```python
from build123d import *

# Parameters (mm, degrees)
SKETCH_1_R          = 15.75
SKETCH_1_R_2        = 1.6
EXTRUDE_1_DEPTH     = 3
EXTRUDE_2_DEPTH     = 3
SKETCH_3_W          = 20
SKETCH_3_H          = 31.5
EXTRUDE_3_DEPTH     = 5
SKETCH_4_R          = 1.25
CUT_EXTRUDE_1_DEPTH = 10


with BuildPart() as part:
    # 草图1 → 凸台-拉伸1 (new body)
    with BuildSketch(Plane(origin=(0, 0, 0), x_dir=(1, 0, 0), z_dir=(0, 1, 0))):
        Circle(SKETCH_1_R)
        with Locations((0, 8)):
            Circle(SKETCH_1_R_2, mode=Mode.SUBTRACT)
        with Locations((8, 0)):
            Circle(SKETCH_1_R_2, mode=Mode.SUBTRACT)
        with Locations((0, -8)):
            Circle(SKETCH_1_R_2, mode=Mode.SUBTRACT)
        with Locations((-8, 0)):
            Circle(SKETCH_1_R_2, mode=Mode.SUBTRACT)
    extrude(amount=EXTRUDE_1_DEPTH)

    # 草图2 → 凸台-拉伸2 (add)
    with BuildSketch(Plane.XZ):
        with BuildLine():
            Line((0, 15.75), (55, 15.75))
            Line((55, 15.75), (55, -15.75))
            Line((55, -15.75), (0, -15.75))
            ThreePointArc((0, -15.75), (15.75, 0), (0, 15.75))
        make_face()
    extrude(amount=-EXTRUDE_2_DEPTH)

    # 草图3 → 凸台-拉伸3 (add)
    with BuildSketch(Plane.XZ):
        with Locations((45, 0)):
            Rectangle(SKETCH_3_W, SKETCH_3_H)
    extrude(amount=-EXTRUDE_3_DEPTH)

    # 草图4 → 切除-拉伸1 (cut)
    with BuildSketch(Plane(origin=(0, 5, 0), x_dir=(1, 0, 0), z_dir=(0, 1, 0))):
        with Locations((45, 4.5)):
            Circle(SKETCH_4_R)
        with Locations((45, -4.5)):
            Circle(SKETCH_4_R)
    extrude(amount=-CUT_EXTRUDE_1_DEPTH, mode=Mode.SUBTRACT)


solid = part.part
```
Input: part model. Units: mm. Frame: model coordinates. A direction names the side the tool comes from. Coordinates: 2 decimals unless noted, no trailing zeros. Write each loop counter-clockwise with the first axis right and the second up, starting at its lowest first coordinate (ties: lowest second). Pieces come first, ordered by that corner, then holes.
1) Section D-D on z = 4.5. Output: boundary loops of the cut face in (x, y), and give its area (3 significant figures).
2) Set-up query: faces 5 (the flat face through (10, 3, 0)), 6 (the flat face through (33, 2, 15.75)). Return all of +Z, -Z, +X, -X, +Y, -Y with unobstructed straight access to the full face (end or side cutting, diameter ignored); none if empty.
3) Section B-B on y = 1.45. Output: boundary loops of the cut face in (x, z), and give its area (3 significant figures).
4) Section C-C on x = 8. Output: boundary loops of the cut face in (y, z), and give its area (3 significant figures).
5) Pin query (flat end, axial travel): pin 1 Ø3 at (x, z) = (45, -4.5) entering from +Y; pin 2 Ø4 at (x, z) = (0, 8) entering from +Y; pin 3 Ø1 at (y, z) = (4, 1.5) entering from -X; pin 4 Ø2 at (y, z) = (3.5, 4) entering from -X. Return the tip coordinate at first contact, or that it passes through.
6) Mould query, pull axis Z, two halves, no side actions, for faces 1 (the flat face through (34, 2, -15.75)), 2 (the cylindrical face through (-15.746, 1.479, -0.346)), 3 (the cylindrical face through (44.01, 2.54, 5.26)), 4 (the flat face through (55, 2, 0)). Classes: pulls with the +Z half, pulls with the -Z half, needs draft (parallel to the pull), parting line crosses it, or undercut.
7) Material intervals for line 1 along Z through (x, y) = (45, 2.7); line 2 along X through (y, z) = (0.8, 0); line 3 along Z through (x, y) = (0, 1.35), sorted ascending.
8) Section A-A on x = 45. Output: boundary loops of the cut face in (y, z).
Check result:
1. outline: (-15.09, 0) - (43.75, 0) - (43.75, 5) - (35, 5) - (35, 3) - (-15.09, 3) - close; (46.25, 0) - (55, 0) - (55, 5) - (46.25, 5) - close
1. area: 238 mm2
2. face 5: +Z, -Z, -X, +Y
2. face 6: +Z, +X, -X, +Y, -Y
3. outline: (0, -15.75) - (55, -15.75) - (55, 15.75) - (0, 15.75) arc R15.75 ccw to start; hole circle Ø3.2 at (-8, 0); hole circle Ø3.2 at (0, -8); hole circle Ø3.2 at (0, 8); hole circle Ø3.2 at (8, 0); hole circle Ø2.5 at (45, -4.5); hole circle Ø2.5 at (45, 4.5)
3. area: 2,080 mm2
4. outline: (0, -15.75) - (3, -15.75) - (3, -1.6) - (0, -1.6) - close; (0, 1.6) - (3, 1.6) - (3, 15.75) - (0, 15.75) - close
4. area: 84.9 mm2
5. pin 1: stops at y = 5
5. pin 2: stops at y = 3
5. pin 3: stops at x = 35
5. pin 4: stops at x = -15.44
6. face 1: pulls with the -Z half
6. face 2: parting line crosses it
6. face 3: undercut
6. face 4: needs draft
7. line 1: z = -15.75 to -5.75, -3.25 to 3.25, 5.75 to 15.75
7. line 2: x = -15.75 to -9.6, -6.4 to 6.4, 9.6 to 55
7. line 3: z = -15.75 to -9.6, -6.4 to 6.4, 9.6 to 15.75
8. outline: (0, -15.75) - (5, -15.75) - (5, -5.75) - (0, -5.75) - close; (0, -3.25) - (5, -3.25) - (5, 3.25) - (0, 3.25) - close; (0, 5.75) - (5, 5.75) - (5, 15.75) - (0, 15.75) - close
